from build123d import *

# Parameters (mm, degrees)
BOSS_EXTRUDE3_DEPTH = 0.8
FILLET2_R           = 3
SKETCH2_R           = 1
CUT_EXTRUDE1_DEPTH  = 79.859431903


with BuildPart() as part:
    # Sketch1 → Boss-Extrude3 (new, symmetric)
    with BuildSketch(Plane.XY):
        with BuildLine():
            ThreePointArc((5.75, 78), (8.53922468, 72.493261963), (9.5, 66.395651864))
            Line((9.5, 66.395651864), (9.5, 46.645651864))
            Line((9.5, 46.645651864), (4.5, 43.144614173))
            Line((4.5, 43.144614173), (4.5, 27.994614173))
            Line((4.5, 27.994614173), (6.3, 26.955383689))
            Line((6.3, 26.955383689), (9.165788003, 18.951905633))
            Line((9.165788003, 18.951905633), (11.5, 17.994614173))
            Line((11.5, 17.994614173), (10, 0))
            Line((10, 0), (0, 0))
            Line((0, 0), (0, 6))
            Line((0, 6), (3.006461475, 66.80874217))
            ThreePointArc((3.006461475, 66.80874217), (3.842195438, 72.535780218), (5.75, 78))
        make_face()
        with BuildLine():
            ThreePointArc((1.944453421, 45.328548769), (-2.087316609, 40.592191664), (1.45758967, 35.481234056))
            Line((1.45758967, 35.481234056), (1.944453421, 45.328548769))
        make_face()
    extrude(amount=BOSS_EXTRUDE3_DEPTH, both=True)

    # Fillet2
    fillet2_edges = [part.edges().sort_by_distance(p)[0] for p in [
        (10, 0, 0),
    ]]
    fillet(fillet2_edges, radius=FILLET2_R)

    # Sketch2 → Cut-Extrude1 (cut, through all)
    with BuildSketch(Plane.XY.offset(0.8)):
        with Locations((6.5, 5.01349848)):
            Circle(SKETCH2_R)
    extrude(amount=-CUT_EXTRUDE1_DEPTH, mode=Mode.SUBTRACT)


solid = part.part
Source: CAD feature listing. Evaluate the final solid. Frame: model axes, mm. A direction names the side the tool comes from. Give positions to 0.01 mm unless a question says otherwise; leave off trailing zeros. Order: outer loops, then holes, each group sorted by start corner. A loop starts at its lowest first (then second) coordinate and runs counter-clockwise, first axis right, second up. Notation, with made-up numbers: (-40, -29.75) -> (-27, -29.75) arc R19 ccw to (-27, -3.75) -> close; hole circle Ø11 at (16.5, 22). An arc over 180 degrees is marked (long way). Write item = value, one per line.
Item 1: Section query B-B (x = 3.75). Output: boundary loops of the cut face in (y, z).
Check result:
outline = (0, -0.8) -> (72.15, -0.8) -> (72.15, 0.8) -> (0, 0.8) -> close
Item 2: Set-up query: faces 1 (the face through (0, 3, 0)), 2 (the face through (5.39, 27.48, 0.01)), 3 (the face through (10.874, 10.479, 0.011)), 4 (the face through (0.72, 20.53, 0.01)), 5 (the face through (9.5, 57, 0)). Return all of +Z, -Z, +X, -X, +Y, -Y with unobstructed straight access to the full face (end or side cutting, diameter ignored); none if empty.
Check result:
face_1 = +Z, -Z, -X, -Y
face_2 = +Z, -Z, +X
face_3 = +Z, -Z, +X, -Y
face_4 = +Z, -Z, -X
face_5 = +Z, -Z, +X, +Y
Item 3: Contact query for flat-ended pins moving along their axis: pin 1 (3 mm diameter, centred on x = 6.5, y = 5.01, fed in from -Z); pin 2 (0.5 mm diameter, centred on y = 61, z = -0.5, fed in from +X); pin 3 (0.8 mm diameter, centred on y = 4, z = 0, fed in from -X); pin 4 (0.8 mm diameter, centred on y = 33.5, z = 0, fed in from +X). Output: stop coordinate, or through.
Check result:
pin_1 = -0.8
pin_2 = 9.5
pin_3 = 0
pin_4 = 4.5
Item 4: Section query A-A (z = -0.4). Output: boundary loops of the cut face in (x, y), then the cut area to 3 significant figures.
Check result:
outline = (0, 0) -> (7.24, 0) arc R3 ccw to (10.23, 2.75) -> (11.5, 17.99) -> (9.17, 18.95) -> (6.3, 26.96) -> (4.5, 27.99) -> (4.5, 43.14) -> (9.5, 46.65) -> (9.5, 66.4) arc R19.83 ccw to (5.75, 78) arc R30.35 ccw to (3.01, 66.81) -> (1.94, 45.33) arc R5.1 ccw to (1.46, 35.48) -> (0, 6) -> close; hole circle Ø2 at (6.5, 5.01)
area = 534 mm²
Item 5: Ray query, probe 1 along X at (y, z) = (67, -0.6); probe 2 along Y at (x, z) = (5.25, 0.05); probe 3 along X at (y, z) = (14, 0.6). Return the intervals inside material, ascending.
Check result:
probe_1 = 3.02 to 9.49
probe_2 = 0 to 27.56, 43.67 to 76.85
probe_3 = 0.4 to 11.17
Item 6: Section query C-C (y = 52). Output: boundary loops of the cut face in (x, z).
Check result:
outline = (2.27, -0.8) -> (9.5, -0.8) -> (9.5, 0.8) -> (2.27, 0.8) -> close
Item 7: Mould query, pull axis Y, two halves, no side actions, for faces 6 (the face through (9.248, 0.771, -0.011)), 7 (the face through (3, 40, 0.8)), 8 (the face through (3.823, 72.457, 0.011)), 9 (the face through (7.713, 23.01, 0.011)). Classes: +Y half, -Y half, draft (parallel to the pull), parting line (faces both ways), or undercut.
Check result:
face_6 = -Y half
face_7 = draft
face_8 = +Y half
face_9 = undercut
